Geometry: see drawing. Coordinates: mm, zero at the bounding-box minimum. Round coordinates to 2 decimals unless told otherwise and drop trailing zeros. Loops run counter-clockwise (first coordinate to the right, second up) from the corner with the lowest first, then second, coordinate; pieces in that order, holes last. Notation, with made-up numbers: (35.5, -27) -> (65.5, -27) arc R21 cw to (65.5, -8) -> close; hole circle Ø3 at (57.25, -19.5). An arc over 180 degrees is marked (long way). Write item = value, one per line.
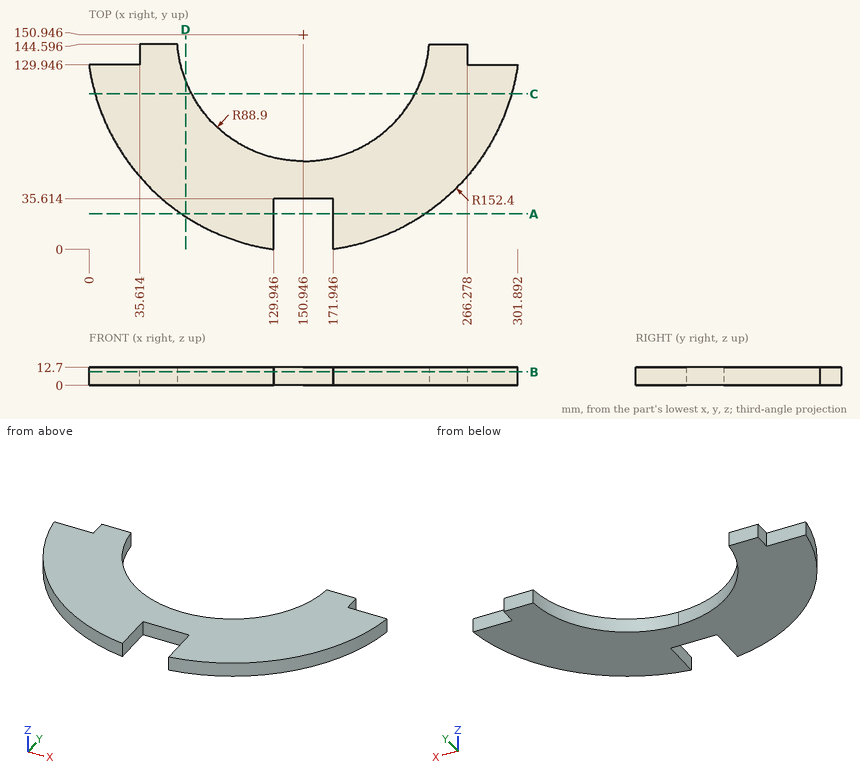
1. Section query C-C (y = 109.5). Return the cut outline in (x, z).
Evaluation:
outline = (4.29, 0) -> (72.3, 0) -> (72.3, 12.7) -> (4.29, 12.7) -> close; (229.59, 0) -> (297.6, 0) -> (297.6, 12.7) -> (229.59, 12.7) -> close
2. Section query D-D (x = 68). Return the cut outline in (y, z).
Evaluation:
outline = (23.1, 0) -> (118.96, 0) -> (118.96, 12.7) -> (23.1, 12.7) -> close
3. Contact query for flat-ended pins moving along their axis: pin 1 Ø4 at (x, z) = (289.5, 7.5) entering from +Y; pin 2 Ø4 at (y, z) = (137.5, 8.5) entering from +X; pin 3 Ø2 at (y, z) = (75.5, 1.5) entering from -X. Output: stop coordinate, or through.
Evaluation:
pin_1 = 129.95
pin_2 = 266.28
pin_3 = 17.97
4. Line query: probe 1 along Y at (x, z) = (150.5, 7.75) (1 decimal); probe 2 along X at (y, z) = (84.5, 9.75) (1 decimal); probe 3 along X at (y, z) = (21.5, 9) (1 decimal). Output: solid intervals per line, ascending. Write a range as from..to.
Evaluation:
probe_1 = 35.6..62
probe_2 = 13.8..91.9, 210..288.1
probe_3 = 70.5..129.9, 171.9..231.4
5. Section query B-B (z = 9.5). Return the cut outline in (x, y) (1 decimal), then the cut area to 3 significant figures.
Evaluation:
outline = (0, 129.9) arc R152.4 ccw to (129.9, 0) -> (129.9, 35.6) -> (171.9, 35.6) -> (171.9, 0) arc R152.4 ccw to (301.9, 129.9) -> (266.3, 129.9) -> (266.3, 144.6) -> (239.6, 144.6) arc R88.9 cw to (62.3, 144.6) -> (35.6, 144.6) -> (35.6, 129.9) -> close
area = 20,700 mm²
6. Section query A-A (y = 25). Return the cut outline in (x, z), then the cut area to 3 significant figures.
Evaluation:
outline = (65.14, 0) -> (129.95, 0) -> (129.95, 12.7) -> (65.14, 12.7) -> close; (171.95, 0) -> (236.76, 0) -> (236.76, 12.7) -> (171.95, 12.7) -> close
area = 1,650 mm²
